The model under review builds one solid part; all positions refer to its coordinate system, in mm. Face numbers are marked on the shaded views. A direction names the side the tool comes from. Round coordinates to 2 decimals unless told otherwise and drop trailing zeros. Order: outer loops, then holes, each group sorted by start corner. A loop starts at its lowest first (then second) coordinate and runs counter-clockwise, first axis right, second up. Notation, with made-up numbers: M 18,63.5 L 45,63.5 A27 cw 45,100.5 Z; hole C 35.25,6 d11. An arc over 180 degrees is marked long. Use a Markdown table: item, result. Add a question column.
1. To check wall thickness, follow probe 1 along X at (y, z) = (-23.5, 6); probe 2 along Y at (x, z) = (0.25, 2.25); probe 3 along Y at (x, z) = (1, 1). State the ranges of each line that lie inside material, in increasing order.
2. For the marked faces 1, 2 and 3, list the 3-axis set-ups (+Z, -Z, +X, -X, +Y, -Y) from which the entire face can be reached by the end or side of a thin tool; tool diameter is ignored.
3. Insertion check: P1, Ø1, axis at y = 4.5, z = 5, coming from the +X side; P2, Ø1, axis at y = -21, z = 1, coming from the -X side; P3, Ø1.1, axis at x = -4.5, z = 2, coming from the -Y side. Each pin has a flat end and moves straight along its axis. Give the tip position at first contact, or say it passes through.
4. Consider section B-B on x = -1.5. State the section outline as (y, z) points.
5. Consider section A-A on z = 3.5. State the section outline as (x, y) points.
6. Consider section D-D on z = 5.25. State the section outline as (x, y) points.
7. Consider section C-C on y = -19. State the section outline as (x, z) points, then the cut area to 3 significant figures.
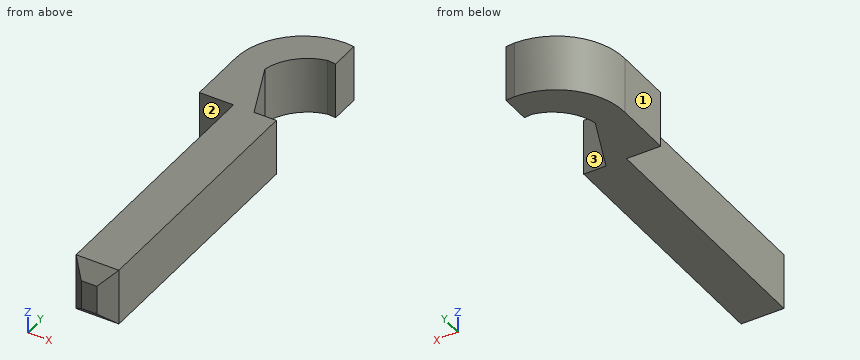
from build123d import *

# Parameters (mm, degrees)
F1_DEPTH = 6.2992
F2_SIZE  = 1.524


with BuildPart() as f1:
    # F0 (on Top) → F1 (new body)
    with BuildSketch(Plane.XY):
        with BuildLine():
            Line((-2.018026, 1.86154), (-2.018026, -28.11046))
            Line((-2.018026, -28.11046), (1.791974, -28.11046))
            Line((1.791974, -28.11046), (2.757174, -28.11046))
            Line((2.757174, -28.11046), (2.757174, 1.86154))
            Line((2.757174, 1.86154), (1.791974, 1.86154))
            Line((1.791974, 1.86154), (0.267974, 1.86154))
            Line((0.267974, 1.86154), (-2.526026, 8.33854))
            ThreePointArc((-2.526026, 8.33854), (-1.007509, 11.138022), (1.791974, 12.65654))
            Line((1.791974, 12.65654), (2.757174, 12.573544))
            Line((2.757174, 12.573544), (2.757174, 15.875544))
            Line((2.757174, 15.875544), (1.791974, 15.95854))
            ThreePointArc((1.791974, 15.95854), (-3.59618, 13.726694), (-5.828026, 8.33854))
            Line((-5.828026, 8.33854), (-5.828026, 1.86154))
            Line((-5.828026, 1.86154), (-2.018026, 1.86154))
        make_face()
    extrude(amount=F1_DEPTH)

    # F2
    f2_edges = [f1.edges().sort_by_distance(p)[0] for p in [
        (0.369574, -28.11046, 6.2992),
        (-2.018026, -28.11046, 3.1496),
        (2.757174, -28.11046, 3.1496),
        (0.369574, -28.11046, 0),
    ]]
    chamfer(f2_edges, length=F2_SIZE)


solid = f1.part
Answer block:
| question | item | result |
|---|---|---|
| 1 | probe 1 | -2.02 to 2.76 |
| 1 | probe 2 | -28.11 to 1.9, 12.08 to 15.8 |
| 1 | probe 3 | -27.59 to 1.86, 12.43 to 15.92 |
| 2 | face 1 | +Z, -Z, -X, +Y, -Y |
| 2 | face 2 | +Z, -Z, -X, -Y |
| 2 | face 3 | +Z, -Z, +X |
| 3 | P1 | x = -0.65 |
| 3 | P2 | x = -2.02 |
| 3 | P3 | y = 1.86 |
| 4 | outline | M -27.1,0.52 L -26.59,0 L 5.96,0 L 5.96,6.3 L -26.59,6.3 L -27.1,5.78 Z; M 10.57,0 L 15.21,0 L 15.21,6.3 L 10.57,6.3 Z |
| 5 | outline | M -5.83,1.86 L -2.02,1.86 L -2.02,-26.59 L -0.49,-28.11 L 1.23,-28.11 L 2.76,-26.59 L 2.76,1.86 L 0.27,1.86 L -2.53,8.34 A5.6 cw 1.79,12.66 L 2.76,12.57 L 2.76,15.88 L 1.79,15.96 A7.62 ccw -5.83,8.34 Z |
| 6 | outline | M -5.83,1.86 L -2.02,1.86 L -2.02,-26.59 L -0.97,-27.64 L 1.71,-27.64 L 2.76,-26.59 L 2.76,1.86 L 0.27,1.86 L -2.53,8.34 A5.6 cw 1.79,12.66 L 2.76,12.57 L 2.76,15.88 L 1.79,15.96 A7.62 ccw -5.83,8.34 Z |
| 7 | outline | M -2.02,0 L 2.76,0 L 2.76,6.3 L -2.02,6.3 Z |
| 7 | area | 30.1 mm^2 |
